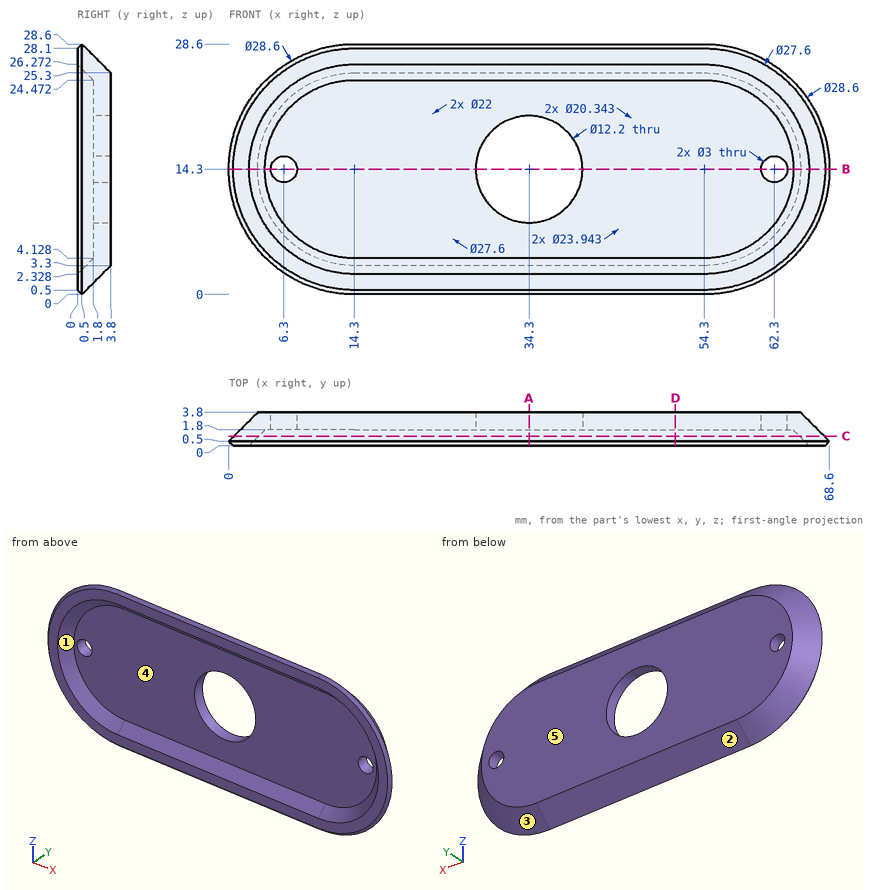
Design review of the part shown in the three views and the two pictorial views. Dimensions are in mm from the part's minimum x, y and z. A direction names the side the tool comes from. Coordinates: 2 decimals unless noted, no trailing zeros. Order: outer loops, then holes, each group sorted by start corner. A loop starts at its lowest first (then second) coordinate and runs counter-clockwise, first axis right, second up.
Item 1: Take a section at A-A, the plane x = 34.3. Write out the cut boundary in (y, z).
Item 2: For pin 1 Ø11 at (x, z) = (34.3, 14.3) entering from +Y; pin 2 Ø1.5 at (y, z) = (1, 3.5) entering from -X; pin 3 Ø6 at (x, z) = (32.5, 19.5) entering from -Y; pin 4 Ø2 at (x, y) = (11, 1.5) entering from -Z, all flat-tipped, find the tip position at first contact; note any pin that passes through.
Item 3: Take a section at B-B, the plane z = 14.3. Write out the cut boundary in (x, y), then the cut area to 3 significant figures.
Item 4: For line 1 (X direction, y = 3.2, z = 14.3); line 2 (X direction, y = 2.3, z = 14.3); line 3 (Y direction, x = 47.5, z = 5.25), list the stretches that pass through material, from the lowest coordinate up.
Item 5: For the marked faces 1 and 2, list the 3-axis set-ups (+Z, -Z, +X, -X, +Y, -Y) from which the entire face can be reached by the end or side of a thin tool; tool diameter is ignored.
Item 6: The part is to be moulded in two halves that separate along X. For the marked faces 3, 4 and 5, say which applies: pulls with the +X half, pulls with the -X half, needs draft (parallel to the pull), parting line crosses it, or undercut.
Item 7: Take a section at C-C, the plane y = 1.1. Write out the cut boundary in (x, z).
Item 8: Take a section at D-D, the plane x = 51. Write out the cut boundary in (y, z).
The answers:
1. outline: (0, 0.5) - (0.5, 0) - (3.8, 3.3) - (3.8, 8.2) - (1.8, 8.2) - (1.8, 4.13) - (0, 2.33) - close; (0, 26.27) - (1.8, 24.47) - (1.8, 20.4) - (3.8, 20.4) - (3.8, 25.3) - (0.5, 28.6) - (0, 28.1) - close
2. pin 1: passes through
2. pin 2: stops at x = 4.32
2. pin 3: stops at y = 1.8
2. pin 4: stops at z = 0.36
3. outline: (0, 0.5) - (0.5, 0) - (2.33, 0) - (4.13, 1.8) - (4.8, 1.8) - (4.8, 3.8) - (3.3, 3.8) - close; (7.8, 1.8) - (28.2, 1.8) - (28.2, 3.8) - (7.8, 3.8) - close; (40.4, 1.8) - (60.8, 1.8) - (60.8, 3.8) - (40.4, 3.8) - close; (63.8, 1.8) - (64.47, 1.8) - (66.27, 0) - (68.1, 0) - (68.6, 0.5) - (65.3, 3.8) - (63.8, 3.8) - close
3. area: 101 mm2
4. line 1: x = 2.7 to 4.8, 7.8 to 28.2, 40.4 to 60.8, 63.8 to 65.9
4. line 2: x = 1.8 to 4.8, 7.8 to 28.2, 40.4 to 60.8, 63.8 to 66.8
4. line 3: y = 1.8 to 3.8
5. face 1: -Y
5. face 2: -Z, +X, -X, +Y
6. face 3: pulls with the +X half
6. face 4: undercut
6. face 5: needs draft
7. outline: (14.3, 0.6) - (54.3, 0.6) arc R13.7 ccw to (54.3, 28) - (14.3, 28) arc R13.7 ccw to start; hole (14.3, 3.43) - (54.3, 3.43) arc R10.87 ccw to (54.3, 25.17) - (14.3, 25.17) arc R10.87 ccw to start
8. outline: (0, 0.5) - (0.5, 0) - (3.8, 3.3) - (3.8, 25.3) - (0.5, 28.6) - (0, 28.1) - (0, 26.27) - (1.8, 24.47) - (1.8, 4.13) - (0, 2.33) - close
